Geometry check sheet. Reference: the model listing, model coordinates, mm. Round coordinates to 2 decimals unless told otherwise and drop trailing zeros. Write each loop counter-clockwise with the first axis right and the second up, starting at its lowest first coordinate (ties: lowest second). Pieces come first, ordered by that corner, then holes. Notation, with made-up numbers: (-14, -37.75) -> (5, -37.75) arc R19 cw to (5, -13.75) -> close; hole circle Ø10 at (17.25, -30.5). An arc over 180 degrees is marked (long way). Put each result on its own line as item: value. Start each with the question number.
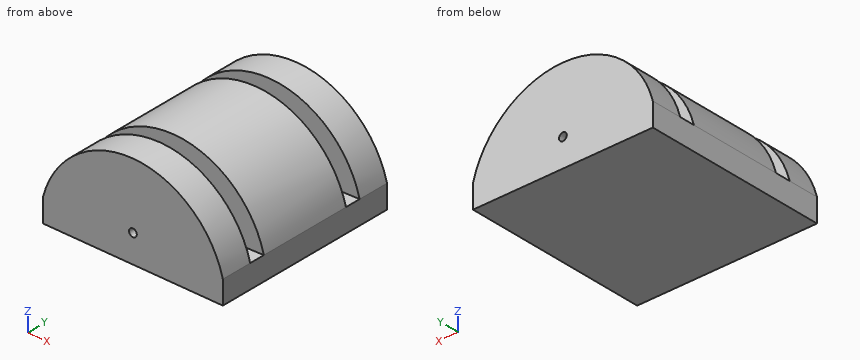
from build123d import *

# Parameters (mm, degrees)
F1_DEPTH = 76.2
F2_START = -38.1
F2_DEPTH = 12.7
F3_R     = 3.175
F4_DEPTH = 152.4


# Not quite as in the source:
# - a pattern or mirror of a feature is missing from the dataset's text; its kind, count and spacing are read off the source's solid


with BuildPart() as f1:
    # F0 (on Front) → F1 (new body, symmetric)
    with BuildSketch(Plane.XZ):
        Polygon((73.7803327453, 0), (73.7803327453, 19.05), (0, 16.51), (-73.7803327453, 19.05), (-73.7803327453, 0), align=None)
        with BuildLine():
            Line((0, 16.51), (73.7803327453, 19.05))
            ThreePointArc((73.7803327453, 19.05), (0, 76.2), (-73.7803327453, 19.05))
            Line((-73.7803327453, 19.05), (0, 16.51))
        make_face()
    extrude(amount=F1_DEPTH, both=True)

    # F0 (on Front) → F2 (cut)
    with BuildSketch(Plane.XZ.offset(F2_START)):
        with BuildLine():
            Line((0, 16.51), (73.7803327453, 19.05))
            ThreePointArc((73.7803327453, 19.05), (0, 76.2), (-73.7803327453, 19.05))
            Line((-73.7803327453, 19.05), (0, 16.51))
        make_face()
    f2 = extrude(amount=-F2_DEPTH, mode=Mode.SUBTRACT)

    # F2_copies: F2 across plane
    add(f2.mirror(Plane(origin=(0, 0, 0), x_dir=(0, 0, -1), z_dir=(0, -1, 0))), mode=Mode.SUBTRACT)

    # F3 (on face) → F4 (cut)
    with BuildSketch(Plane.XZ.offset(76.2)):
        with Locations((0, 22.86)):
            Circle(F3_R)
    extrude(amount=-F4_DEPTH, mode=Mode.SUBTRACT)


solid = f1.part
(1) Go/stop test with flat-tipped pins: pin 1 Ø3 at (y, z) = (-53.5, 39) entering from -X; pin 2 Ø3 at (y, z) = (33.5, 47) entering from +X; pin 3 Ø12 at (x, y) = (-36.5, -15.5) entering from +Z. Record where each tip stops, or that it passes through.
(2) Sectioned sample at A-A (z = 22.86). Record the cut outline in (x, y) (3 decimals), and give its area (3 significant figures).
(3) Sectioned sample at C-C (z = 72). Record the cut outline in (x, y).
(4) Sectioned sample at D-D (x = -48). Record the cut outline in (y, z).
(5) Material ranges on L1, parallel to Y at x = 3.5, z = 61.5; L2, parallel to X at y = 65, z = 22; L3, parallel to Z at x = 45.5, y = 3, recorded low to high. Write a range as from..to.
(6) Sectioned sample at B-B (y = 28). Record the cut outline in (x, z) (3 decimals), and give its area (3 significant figures).
Found:
1. pin 1: x = -66.33
1. pin 2: x = 61.12
1. pin 3: z = 69.83
2. outline: (-72.69, -76.2) -> (-3.175, -76.2) -> (-3.175, -50.8) -> (-72.69, -50.8) -> close; (-72.69, -38.1) -> (-3.175, -38.1) -> (-3.175, 38.1) -> (-72.69, 38.1) -> close; (-72.69, 50.8) -> (-3.175, 50.8) -> (-3.175, 76.2) -> (-72.69, 76.2) -> close; (3.175, -76.2) -> (72.69, -76.2) -> (72.69, -50.8) -> (3.175, -50.8) -> close; (3.175, -38.1) -> (72.69, -38.1) -> (72.69, 38.1) -> (3.175, 38.1) -> close; (3.175, 50.8) -> (72.69, 50.8) -> (72.69, 76.2) -> (3.175, 76.2) -> close
2. area: 17,700 mm2
3. outline: (-24.95, -76.2) -> (24.95, -76.2) -> (24.95, -50.8) -> (-24.95, -50.8) -> close; (-24.95, -38.1) -> (24.95, -38.1) -> (24.95, 38.1) -> (-24.95, 38.1) -> close; (-24.95, 50.8) -> (24.95, 50.8) -> (24.95, 76.2) -> (-24.95, 76.2) -> close
4. outline: (-76.2, 0) -> (76.2, 0) -> (76.2, 59.18) -> (50.8, 59.18) -> (50.8, 18.16) -> (38.1, 18.16) -> (38.1, 59.18) -> (-38.1, 59.18) -> (-38.1, 18.16) -> (-50.8, 18.16) -> (-50.8, 59.18) -> (-76.2, 59.18) -> close
5. L1: -76.2..-50.8, -38.1..38.1, 50.8..76.2
5. L2: -72.96..-3.06, 3.06..72.96
5. L3: 0..61.12
6. outline: (-73.78, 0) -> (73.78, 0) -> (73.78, 19.05) arc R76.2 ccw to (-73.78, 19.05) -> close; hole circle Ø6.35 at (0, 22.86)
6. area: 9,030 mm2
